The model under review builds one solid part; all positions refer to its coordinate system, in mm. A direction names the side the tool comes from. Give positions to 0.01 mm unless a question says otherwise; leave off trailing zeros. Write each loop counter-clockwise with the first axis right and the second up, starting at its lowest first coordinate (ties: lowest second). Pieces come first, ordered by that corner, then holes. Notation, with made-up numbers: (53.25, 28) - (87.25, 28) arc R12 ccw to (87.25, 50) - close; hole circle Ø3 at (58, 67). An arc over 180 degrees is marked (long way). Write item = value, one per line.
```python
from build123d import *

# Parameters (mm, degrees)
SM_BASE_FLANGE_1_DEPTH   = 41
SKETCH_9_R               = 2.5
SKETCH_9_R_2             = 2
CUT_EXTRUDE_4_DEPTH      = 61.6465168
CUT_EXTRUDE_5_DEPTH      = 78.103826105
CUT_EXTRUDE_5_DEPTH_BACK = 78.103826105
SKETCH_10_R              = 2


# Sheet-metal steps are written as plain solids
with BuildPart() as part:
    # Sketch 1 → Базовая кромка1 (new body)
    with BuildSketch(Plane.XY):
        with BuildLine():
            Line((-25, 30), (-25, 1))
            ThreePointArc((-25, 1), (-24.707106781, 0.292893219), (-24, 0))
            Line((-24, 0), (24, 0))
            ThreePointArc((24, 0), (24.707106781, 0.292893219), (25, 1))
            Line((25, 1), (25, 30))
            Line((25, 30), (29, 30))
            Line((29, 30), (29, 1))
            ThreePointArc((29, 1), (27.535533906, -2.535533906), (24, -4))
            Line((24, -4), (-24, -4))
            ThreePointArc((-24, -4), (-27.535533906, -2.535533906), (-29, 1))
            Line((-29, 1), (-29, 30))
            Line((-29, 30), (-25, 30))
        make_face()
    extrude(amount=SM_BASE_FLANGE_1_DEPTH)

    # Эскиз9 → Вырез-Вытянуть4 (cut, through all)
    with BuildSketch(Plane.XZ.offset(4)):
        with Locations((-18, 20.5)):
            Circle(SKETCH_9_R)
        with Locations((-9, 36.088457268)):
            Circle(SKETCH_9_R)
        with Locations((9, 36.088457268)):
            Circle(SKETCH_9_R)
        with Locations((18, 20.5)):
            Circle(SKETCH_9_R)
        with Locations((9, 4.911542732)):
            Circle(SKETCH_9_R)
        with Locations((-9, 4.911542732)):
            Circle(SKETCH_9_R)
        with Locations((0, 5)):
            Circle(SKETCH_9_R_2)
        with Locations((-13.423393759, 12.75)):
            Circle(SKETCH_9_R_2)
        with Locations((-13.423393759, 28.25)):
            Circle(SKETCH_9_R_2)
        with Locations((0, 36)):
            Circle(SKETCH_9_R_2)
        with Locations((13.423393759, 28.25)):
            Circle(SKETCH_9_R_2)
        with Locations((13.423393759, 12.75)):
            Circle(SKETCH_9_R_2)
    extrude(amount=-CUT_EXTRUDE_4_DEPTH, mode=Mode.SUBTRACT)

    # Эскиз10 → Вырез-Вытянуть5 (cut, two sides: drawn at the far end of the back side and taken through both)
    with BuildSketch(Plane(origin=(29, 0, 0), x_dir=(0, 0, -1), z_dir=(1, 0, 0)).offset(-CUT_EXTRUDE_5_DEPTH_BACK)):
        with Locations((-33, 25)):
            Circle(SKETCH_10_R)
        with Locations((-20.5, 25)):
            Circle(SKETCH_10_R)
        with Locations((-8, 25)):
            Circle(SKETCH_10_R)
        with Locations((-20.5, 12.5)):
            Circle(SKETCH_10_R)
    extrude(amount=CUT_EXTRUDE_5_DEPTH + CUT_EXTRUDE_5_DEPTH_BACK, mode=Mode.SUBTRACT)


solid = part.part
```
1. Insertion check: P1, Ø8, axis at x = 9, z = 36.09, coming from the +Y side. The pin has a flat end and moves straight along its axis. Give the tip position at first contact, or say it passes through.
Findings below:
P1 = 0
2. Draft analysis for pull direction Y (two halves, no side actions). For faces 1 (the flat face through (0, -4, 20)), 2 (the cylindrical face through (-27, 23.8, 22.1)), 3 (the flat face through (-25, 16, 20)), 4 (the flat face through (-27, 30, 20)), state which applies: +Y half, -Y half, draft (parallel to the pull), parting line (faces both ways), or undercut.
Findings below:
face_1 = -Y half
face_2 = undercut
face_3 = draft
face_4 = +Y half
3. For line 1 (Z direction, x = -9, y = -2); line 2 (Z direction, x = 18, y = -1); line 3 (Z direction, x = 25.8, y = 25), list the stretches that pass through material, from the lowest coordinate up. Write a range as from..to.
Findings below:
line_1 = 0..2.41, 7.41..33.59, 38.59..41
line_2 = 0..18, 23..41
line_3 = 0..6, 10..18.5, 22.5..31, 35..41
4. Take a section at D-D on y = 12.5. Give the boundary of the cut face in (x, z).
Findings below:
outline = (-29, 0) - (-25, 0) - (-25, 18.5) - (-29, 18.5) - close; (-29, 22.5) - (-25, 22.5) - (-25, 41) - (-29, 41) - close; (25, 0) - (29, 0) - (29, 18.5) - (25, 18.5) - close; (25, 22.5) - (29, 22.5) - (29, 41) - (25, 41) - close
5. Take a section at A-A on x = 18. Give the boundary of the cut face in (y, z).
Findings below:
outline = (-4, 0) - (0, 0) - (0, 18) - (-4, 18) - close; (-4, 23) - (0, 23) - (0, 41) - (-4, 41) - close
6. Machinability: for faces 5 (the flat face through (0, 0, 20)), 6 (the cylindrical face through (-14.9, -2, 14.1)), which of the approach directions +Z, -Z, +X, -X, +Y, -Y give a long, thin tool a straight path to every point of the face, cutting with its end or side? Answer none if there is none.
Findings below:
face_5 = +Z, -Z, +Y
face_6 = +Y, -Y
7. Take a section at B-B on z = 12.75. Give the boundary of the cut face in (x, y).
Findings below:
outline = (-29, 1) arc R5 ccw to (-24, -4) - (-15.42, -4) - (-15.42, 0) - (-24, 0) arc R1 cw to (-25, 1) - (-25, 30) - (-29, 30) - close; (-11.42, -4) - (11.42, -4) - (11.42, 0) - (-11.42, 0) - close; (15.42, -4) - (24, -4) arc R5 ccw to (29, 1) - (29, 30) - (25, 30) - (25, 1) arc R1 cw to (24, 0) - (15.42, 0) - close
8. Take a section at C-C on y = 7.5. Give the boundary of the cut face in (x, z), and give its area (3 significant figures).
Findings below:
outline = (-29, 0) - (-25, 0) - (-25, 41) - (-29, 41) - close; (25, 0) - (29, 0) - (29, 41) - (25, 41) - close
area = 328 mm²
